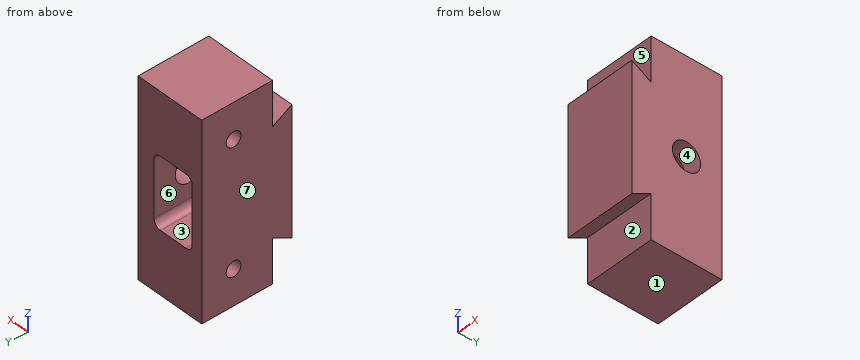
from build123d import *

# Parameters (mm, degrees)
BOSS_EXTRUDE1_DEPTH             = 10
F_8_0MM_DOWEL_HOLE2_D           = 8
F_8_0MM_DOWEL_HOLE2_DEPTH       = 5
TAP_DRILL_FOR_M5X0_8_TAP1_D     = 4.2
TAP_DRILL_FOR_M5X0_8_TAP1_DEPTH = 10
TAP_DRILL_FOR_M5X0_8_TAP1_TIP   = 1.2618073
SKETCH7_OUTSIDE_W               = 34.768
SKETCH7_OUTSIDE_H               = 69.768
SKETCH7_OUTSIDE_W_2             = 20
SKETCH7_OUTSIDE_H_2             = 55
CUT_EXTRUDE1_DEPTH              = 16


with BuildPart() as part:
    # Sketch1 → Boss-Extrude1 (new body, symmetric)
    with BuildSketch(Plane(origin=(0, 0, 0), x_dir=(0, 0, -1), z_dir=(1, 0, 0))):
        Polygon((-55, -20), (-42.5, -20), (-45.5, -25.5), (-9.5, -25.5), (-12.5, -20), (0, -20), (0, 0), (-55, 0), align=None)
    extrude(amount=BOSS_EXTRUDE1_DEPTH, both=True)

    # Ø8.0mm Dowel Hole2
    with Locations(Plane(origin=(10, -10, 27.838852212), x_dir=(0, 0, 1), z_dir=(1, 0, 0))):
        with Locations((0, 0)):
            Hole(F_8_0MM_DOWEL_HOLE2_D / 2, depth=F_8_0MM_DOWEL_HOLE2_DEPTH)

    # Tap Drill for M5x0.8 Tap1
    with Locations(Plane(origin=(-10, -9, 10), x_dir=(0, 0, -1), z_dir=(-1, 0, 0))):
        with Locations((0, 0), (-35, 0)):
            Hole(TAP_DRILL_FOR_M5X0_8_TAP1_D / 2, depth=TAP_DRILL_FOR_M5X0_8_TAP1_DEPTH)
            with Locations((0, 0, -(TAP_DRILL_FOR_M5X0_8_TAP1_DEPTH + TAP_DRILL_FOR_M5X0_8_TAP1_TIP / 2))):  # 118° drill point
                Cone(0, TAP_DRILL_FOR_M5X0_8_TAP1_D / 2, TAP_DRILL_FOR_M5X0_8_TAP1_TIP, mode=Mode.SUBTRACT)

    # Sketch7 outside → Cut-Extrude1 (cut)
    with BuildSketch(Plane(origin=(0, 0, 0), x_dir=(1, 0, 0), z_dir=(0, 1, 0))):
        with Locations((0, -27.5)):
            Rectangle(SKETCH7_OUTSIDE_W, SKETCH7_OUTSIDE_H)
        with Locations((0, -27.5)):
            Rectangle(SKETCH7_OUTSIDE_W_2, SKETCH7_OUTSIDE_H_2, mode=Mode.SUBTRACT)
        with BuildLine():
            Line((3, -17.5), (-5, -17.5))
            ThreePointArc((-5, -17.5), (-6.414213562, -18.085786438), (-7, -19.5))
            Line((-7, -19.5), (-7, -35.5))
            ThreePointArc((-7, -35.5), (-6.414213562, -36.914213562), (-5, -37.5))
            Line((-5, -37.5), (3, -37.5))
            ThreePointArc((3, -37.5), (4.414213562, -36.914213562), (5, -35.5))
            Line((5, -35.5), (5, -19.5))
            ThreePointArc((5, -19.5), (4.414213562, -18.085786438), (3, -17.5))
        make_face()
    extrude(amount=-CUT_EXTRUDE1_DEPTH, mode=Mode.SUBTRACT)


solid = part.part
Build history of the part. All positions in model axes, mm. Face numbers are marked on the shaded views. A direction names the side the tool comes from. Round coordinates to 2 decimals unless told otherwise and drop trailing zeros. Write each loop counter-clockwise with the first axis right and the second up, starting at its lowest first coordinate (ties: lowest second). Pieces come first, ordered by that corner, then holes. Notation, with made-up numbers: (-13.5, 36) -> (23.5, 36) arc R15 cw to (23.5, 46) -> close; hole circle Ø4 at (13, 34). An arc over 180 degrees is marked (long way). Write item = value, one per line.
(1) Tool access for the marked faces 1, 2, 3 and 4: list every direction of +Z, -Z, +X, -X, +Y, -Y with a clear straight run to the whole face (end or side of a thin tool).
Answer:
face_1 = -Z, +X, -X, +Y, -Y
face_2 = -Z, +X, -X
face_3 = +Y
face_4 = +X
(2) Band-saw the part on D-D (z = 23). Give the cut face in (x, y), then the cut area to 3 significant figures.
Answer:
outline = (-10, -25.5) -> (10, -25.5) -> (10, 0) -> (5, 0) -> (5, -16) -> (-7, -16) -> (-7, 0) -> (-10, 0) -> close
area = 318 mm2
(3) Two-plate mould, pull along X, no slides. Class the marked faces 5, 6 and 7: pulls with the +X half, pulls with the -X half, needs draft (parallel to the pull), parting line crosses it, or undercut.
Answer:
face_5 = needs draft
face_6 = undercut
face_7 = pulls with the -X half
(4) Probe L1, parallel to Z at x = -3.5, y = -9; L2, parallel to Y at x = -2.75, z = 45; L3, parallel to Z at x = -6.5, y = -9. List the from-to ranges inside material, lowest first.
Answer:
L1 = 0 to 7.9, 12.1 to 17.5, 37.5 to 42.9, 47.1 to 55
L2 = -25.5 to -24.58, -20 to -11.1, -6.9 to 0
L3 = 0 to 7.9, 12.1 to 18.18, 36.82 to 42.9, 47.1 to 55
(5) Band-saw the part on C-C (x = 7.75). Give the cut face in (y, z), then the cut area to 3 significant figures.
Answer:
outline = (-25.5, 9.5) -> (-20, 12.5) -> (-20, 0) -> (0, 0) -> (0, 55) -> (-20, 55) -> (-20, 42.5) -> (-25.5, 45.5) -> close; hole circle Ø8 at (-10, 27.84)
area = 1,230 mm2
(6) Band-saw the part on A-A (x = -3.5). Give the cut face in (y, z).
Answer:
outline = (-25.5, 9.5) -> (-20, 12.5) -> (-20, 0) -> (0, 0) -> (0, 17.5) -> (-16, 17.5) -> (-16, 37.5) -> (0, 37.5) -> (0, 55) -> (-20, 55) -> (-20, 42.5) -> (-25.5, 45.5) -> close; hole circle Ø4.2 at (-9, 10); hole circle Ø4.2 at (-9, 45)
(7) Band-saw the part on B-B (z = 28.5). Give the cut face in (x, y), then the cut area to 3 significant figures.
Answer:
outline = (-10, -25.5) -> (10, -25.5) -> (10, -13.94) -> (5, -13.94) -> (5, -16) -> (-7, -16) -> (-7, 0) -> (-10, 0) -> close; (5, -6.06) -> (10, -6.06) -> (10, 0) -> (5, 0) -> close
area = 279 mm2
(8) Flat gauge pins, fed straight in: pin 1 (5 mm diameter, centred on y = -10, z = 27.84, fed in from +X); pin 2 (6 mm diameter, centred on x = 1, z = 31.5, fed in from +Y). Where does each tip first touch, or does it go through?
Answer:
pin_1 = -7
pin_2 = -16
